```python
from build123d import *

# Parameters (mm, degrees)
BOSS_EXTRU_1_DEPTH      = 44
ESQUISSE2_R             = 7
ENL_V_MAT_EXTRU_1_DEPTH = 44
ENL_V_MAT_EXTRU_2_DEPTH = 19
ESQUISSE4_R             = 5.5
ENL_V_MAT_EXTRU_3_DEPTH = 50
ENL_V_START             = -19
ENL_V_MAT_EXTRU_5_DEPTH = 19
ENL_V_START_2           = -32
ENL_V_MAT_EXTRU_8_DEPTH = 32
BOSS_EXTRU_3_START      = -8
BOSS_EXTRU_3_DEPTH      = 8
ESQUISSE15_R            = 5.5
ENL_V_MAT_EXTRU_9_DEPTH = 44


with BuildPart() as part:
    # Esquisse1 → Boss.-Extru.1 (new body)
    with BuildSketch(Plane.XY):
        with BuildLine():
            Line((69.055498862, 42.585779817), (98.055498862, 42.585779817))
            Line((98.055498862, 42.585779817), (103.055498862, 37.585779817))
            Line((103.055498862, 37.585779817), (103.055498862, 18.585779817))
            Line((103.055498862, 18.585779817), (74.055498862, -15.414220183))
            Line((74.055498862, -15.414220183), (68.352478915, -15.414220183))
            ThreePointArc((68.352478915, -15.414220183), (64.19229693, -9.118662105), (61.797161375, -1.962930743))
            ThreePointArc((61.797161375, -1.962930743), (60.309086392, 2.242265049), (56.055498862, 3.585779817))
            Line((56.055498862, 3.585779817), (24.055498862, 3.585779817))
            Line((24.055498862, 3.585779817), (17.055498862, 10.585779817))
            Line((17.055498862, 10.585779817), (17.055498862, 28.585779817))
            Line((17.055498862, 28.585779817), (24.055498862, 35.585779817))
            Line((24.055498862, 35.585779817), (31.055498862, 35.585779817))
            Line((31.055498862, 35.585779817), (52.765077496, 31.757795364))
            ThreePointArc((52.765077496, 31.757795364), (62.410764196, 34.914360395), (69.055498862, 42.585779817))
        make_face()
    extrude(amount=BOSS_EXTRU_1_DEPTH)

    # Esquisse2 → Enlèv. mat.-Extru.1 (cut)
    with BuildSketch(Plane.XY.offset(44)):
        with Locations((31.055498862, 17.585779817)):
            Circle(ESQUISSE2_R)
    extrude(amount=-ENL_V_MAT_EXTRU_1_DEPTH, mode=Mode.SUBTRACT)

    # Esquisse3 → Enlèv. mat.-Extru.2 (cut)
    with BuildSketch(Plane.XY.offset(44)):
        Polygon((17.055498862, 28.585779817), (17.055498862, 10.585779817), (24.055498862, 3.585779817), (51.055498862, 3.585779817), (51.055498862, 32.059240202), (31.055498862, 35.585779817), (24.055498862, 35.585779817), align=None)
    extrude(amount=-ENL_V_MAT_EXTRU_2_DEPTH, mode=Mode.SUBTRACT)

    # Esquisse4 → Enlèv. mat.-Extru.3 (cut)
    with BuildSketch(Plane.XY.offset(44)):
        with Locations((89.055498862, 28.585779817)):
            Circle(ESQUISSE4_R)
    extrude(amount=-ENL_V_MAT_EXTRU_3_DEPTH, mode=Mode.SUBTRACT)

    # Esquisse10 → Enlèv. mat.-Extru.5 (cut)
    with BuildSketch(Plane.XY.offset(44).offset(ENL_V_START)):
        with BuildLine():
            Line((56.055498862, 3.585779817), (90.261381215, 3.585779817))
            Line((90.261381215, 3.585779817), (74.055498862, -15.414220183))
            Line((74.055498862, -15.414220183), (68.352478915, -15.414220183))
            ThreePointArc((68.352478915, -15.414220183), (64.19229693, -9.118662105), (61.797161375, -1.962930743))
            ThreePointArc((61.797161375, -1.962930743), (60.047831429, 1.971925154), (56.055498862, 3.585779817))
        make_face()
    extrude(amount=ENL_V_MAT_EXTRU_5_DEPTH, mode=Mode.SUBTRACT)

    # Esquisse13 → Enlèv. mat.-Extru.8 (cut)
    with BuildSketch(Plane.XY.offset(44).offset(ENL_V_START_2)):
        with BuildLine():
            Line((69.055498862, 42.585779817), (98.055498862, 42.585779817))
            Line((98.055498862, 42.585779817), (103.055498862, 37.585779817))
            Line((103.055498862, 37.585779817), (103.055498862, 18.585779817))
            Line((103.055498862, 18.585779817), (92.820204745, 6.585779817))
            ThreePointArc((92.820204745, 6.585779817), (74.207332122, 17.1537679), (63.456424114, 35.661587231))
            ThreePointArc((63.456424114, 35.661587231), (66.667333439, 38.791037909), (69.055498862, 42.585779817))
        make_face()
    extrude(amount=ENL_V_MAT_EXTRU_8_DEPTH, mode=Mode.SUBTRACT)

    # Esquisse14 → Boss.-Extru.3 (add)
    with BuildSketch(Plane.XY.offset(44).offset(BOSS_EXTRU_3_START)):
        with BuildLine():
            Line((92.820204745, 6.585779817), (103.055498862, 18.585779817))
            Line((103.055498862, 18.585779817), (103.055498862, 37.585779817))
            Line((103.055498862, 37.585779817), (98.055498862, 42.585779817))
            Line((98.055498862, 42.585779817), (69.055498862, 42.585779817))
            ThreePointArc((69.055498862, 42.585779817), (66.667333439, 38.791037909), (63.456424114, 35.661587231))
            ThreePointArc((63.456424114, 35.661587231), (74.207332122, 17.1537679), (92.820204745, 6.585779817))
        make_face()
    extrude(amount=BOSS_EXTRU_3_DEPTH)

    # Esquisse15 → Enlèv. mat.-Extru.9 (cut)
    with BuildSketch(Plane.XY.offset(44)):
        with Locations((89.055498862, 28.585779817)):
            Circle(ESQUISSE15_R)
    extrude(amount=-ENL_V_MAT_EXTRU_9_DEPTH, mode=Mode.SUBTRACT)


solid = part.part
```
The model under review builds one solid part; all positions refer to its coordinate system, in mm. A direction names the side the tool comes from. Round coordinates to 2 decimals unless told otherwise and drop trailing zeros. Loops run counter-clockwise (first coordinate to the right, second up) from the corner with the lowest first, then second, coordinate; pieces in that order, holes last. Notation, with made-up numbers: M 86,87.5 L 137,87.5 A25 ccw 137,104.5 Z; hole C 42,87 d8. An arc over 180 degrees is marked long. Answer as a JSON object with one key per item and string values.
(1) Take a section at C-C on y = 8.5. Give the boundary of the cut face in (x, z), and give its area (3 significant figures).
Resolved:
{"outline": "M 19.14,0 L 94.45,0 L 94.45,12 L 87.15,12 L 87.15,36 L 94.45,36 L 94.45,44 L 51.06,44 L 51.06,25 L 19.14,25 Z", "area": "2,530 mm²"}
(2) Take a section at B-B on z = 15. Give the boundary of the cut face in (x, y), and give its area (3 significant figures).
Resolved:
{"outline": "M 17.06,10.59 L 24.06,3.59 L 56.06,3.59 A5 cw 61.8,-1.96 A29 ccw 68.35,-15.41 L 74.06,-15.41 L 92.82,6.59 A41 cw 63.46,35.66 A19 cw 52.77,31.76 L 31.06,35.59 L 24.06,35.59 L 17.06,28.59 Z; hole C 31.06,17.59 d14", "area": "1,930 mm²"}
(3) Take a section at A-A on x = 85. Give the boundary of the cut face in (y, z), and give its area (3 significant figures).
Resolved:
{"outline": "M -2.58,0 L 24.87,0 L 24.87,12 L 9.48,12 L 9.48,36 L 24.87,36 L 24.87,44 L 3.59,44 L 3.59,25 L -2.58,25 Z; M 32.3,0 L 42.59,0 L 42.59,12 L 32.3,12 Z; M 32.3,36 L 42.59,36 L 42.59,44 L 32.3,44 Z", "area": "927 mm²"}
(4) Tool access review of faces 5 (the flat face through (74, 3.586, 34)), 6 (the cylindrical face through (74.424, 16.941, 23.832)), 7 (the flat face through (51.055, 18, 35)), 8 (the cylindrical face through (34.29, 11.38, 12.68)): name each direction out of +Z, -Z, +X, -X, +Y, -Y from which nothing blocks a thin tool from reaching the whole face with its end or side.
Resolved:
{"face 5": "+Z, +X, -X, -Y", "face 6": "+X, +Y", "face 7": "+Z, -X, +Y, -Y", "face 8": "+Z, -Z"}
(5) To check wall thickness, follow line 1 along Z through (x, y) = (25, 27.5); line 2 along Y through (x, z) = (71.5, 41.5); line 3 along Y through (x, z) = (37, 7). State the ranges of each line that lie inside material, in increasing order.
Resolved:
{"line 1": "0 to 25", "line 2": "3.59 to 42.59", "line 3": "3.59 to 13.89, 21.28 to 34.54"}
(6) Draft analysis for pull direction Y (two halves, no side actions). For faces 1 (the flat face through (20.6, 7.04, 12.32)), 2 (the flat face through (84, 42.586, 40)), 3 (the cylindrical face through (94.3, 30.24, 6.08)), 4 (the flat face through (38, 23, 25)), state which applies: released by +Y, released by -Y, zero draft, split by the parting line, or undercut.
Resolved:
{"face 1": "released by -Y", "face 2": "released by +Y", "face 3": "undercut", "face 4": "zero draft"}
(7) Clearance check with flat-ended pins moving along their axes: P1, Ø5, axis at x = 36.5, z = 19.5, coming from the +Y side; P2, Ø11, axis at x = 92, y = 27.5, coming from the +Z side; P3, Ø9.5, axis at x = 36, z = 11.5, coming from the -Y side; P4, Ø10, axis at y = 34.5, z = 23.5, coming from the -X side. State where each tip first meets the part, or that it passes through.
Resolved:
{"P1": "y = 35.07", "P2": "z = 44", "P3": "y = 3.59", "P4": "x = 17.97"}
(8) Take a section at D-D on x = 97. Give the boundary of the cut face in (y, z).
Resolved:
{"outline": "M 11.49,0 L 42.59,0 L 42.59,12 L 11.49,12 Z; M 11.49,36 L 42.59,36 L 42.59,44 L 11.49,44 Z"}
